Design review of the part built by this model. Coordinates are the model's own, in mm. Give positions to 0.01 mm unless a question says otherwise; leave off trailing zeros. Write each loop counter-clockwise with the first axis right and the second up, starting at its lowest first coordinate (ties: lowest second). Pieces come first, ordered by that corner, then holes. Notation, with made-up numbers: (15.5, 7) -> (32.5, 7) arc R28 cw to (32.5, 36) -> close; hole circle Ø4 at (-31.75, 23). An arc over 180 degrees is marked (long way). Use CSV: the item, a comma, the result in double quotes.
```python
from build123d import *

# Parameters (mm, degrees)
PAD_DEPTH     = 3
SKETCH001_R   = 3
SKETCH001_R_2 = 2
PAD001_DEPTH  = 0.6


with BuildPart() as part:
    # Sketch → Pad (new body, symmetric)
    with BuildSketch(Plane.XZ):
        with BuildLine():
            Line((-65, 0), (65, 0))
            ThreePointArc((65, 0), (66.499997, 0.401922), (67.598072, 1.499993))
            Line((77.598076, 18.820508), (67.598072, 1.499993))
            Line((77.598076, 18.820508), (75, 20.320508))
            Line((75, 20.320508), (65, 3))
            Line((-65, 3), (65, 3))
            Line((-75, 20.320508), (-65, 3))
            Line((-77.598076, 18.820508), (-75, 20.320508))
            Line((-77.598076, 18.820508), (-67.598088, 1.50002))
            ThreePointArc((-67.598088, 1.50002), (-66.50001, 0.40193), (-65, 0))
        make_face()
    extrude(amount=PAD_DEPTH, both=True)

    # Sketch001 → Pad001 (new body)
    with BuildSketch(Plane(origin=(0, 0, 3), x_dir=(-1, 0, 0), z_dir=(0, 0, 1))):
        with Locations((-32, 0)):
            Circle(SKETCH001_R)
        with Locations((-32, 0)):
            Circle(SKETCH001_R_2, mode=Mode.SUBTRACT)
        with Locations((32, 0)):
            Circle(SKETCH001_R)
        with Locations((32, 0)):
            Circle(SKETCH001_R_2, mode=Mode.SUBTRACT)
    extrude(amount=PAD001_DEPTH)


solid = part.part
```
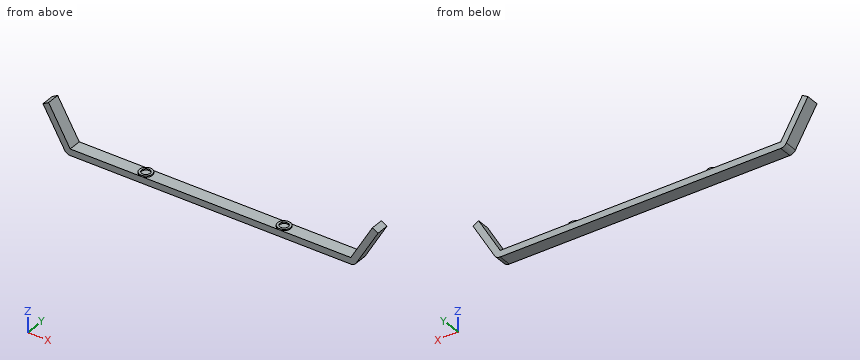
(1) Take a section at C-C (x = 25.5). Write out the cut boundary in (y, z).
Established:
outline,"(-3, 0) -> (3, 0) -> (3, 3) -> (-3, 3) -> close"
(2) Take a section at A-A (y = 0). Write out the cut boundary in (x, z), then the cut area to 3 significant figures.
Established:
outline,"(-77.6, 18.82) -> (-67.6, 1.5) arc R3 ccw to (-65, 0) -> (65, 0) arc R3 ccw to (67.6, 1.5) -> (77.6, 18.82) -> (75, 20.32) -> (65, 3) -> (35, 3) -> (35, 3.6) -> (34, 3.6) -> (34, 3) -> (30, 3) -> (30, 3.6) -> (29, 3.6) -> (29, 3) -> (-29, 3) -> (-29, 3.6) -> (-30, 3.6) -> (-30, 3) -> (-34, 3) -> (-34, 3.6) -> (-35, 3.6) -> (-35, 3) -> (-65, 3) -> (-75, 20.32) -> close"
area,"522 mm2"
(3) Clearance check with flat-ended pins moving along their axes: pin 1 (3 mm diameter, centred on x = -33, y = 0.5, fed in from +Z); pin 2 (3 mm diameter, centred on x = -1, y = -1, fed in from +Z). State where each tip first meets the part, or that it passes through.
Established:
pin 1,"stops at z = 3.6"
pin 2,"stops at z = 3"
(4) For line 1 along Y through (x, z) = (32, 3.4); line 2 along X through (y, z) = (0, 3.1); line 3 along Z through (x, y) = (-10.5, -1.4), list the stretches that pass through material, from the lowest coordinate up. Write a range as [from, to].
Established:
line 1,"y = [-3, -2], [2, 3]"
line 2,"x = [-68.52, -65.06], [-35, -34], [-30, -29], [29, 30], [34, 35], [65.06, 68.52]"
line 3,"z = [0, 3]"
(5) Take a section at B-B (z = 7.25). Write out the cut boundary in (x, y).
Established:
outline,"(-70.92, -3) -> (-67.45, -3) -> (-67.45, 3) -> (-70.92, 3) -> close; (67.45, -3) -> (70.92, -3) -> (70.92, 3) -> (67.45, 3) -> close"
